from build123d import *

# Parameters (mm, degrees)
F0_R     = 3.203715
F1_DEPTH = 3
F2_DEPTH = 25.4
F3_DEPTH = 2
F5_DEPTH = 10


with BuildPart() as f1:
    # F0 (on Top) → F1 (new body)
    with BuildSketch(Plane.XY):
        with BuildLine():
            ThreePointArc((-11.680029, 20.96609), (-17.5, 21.857493), (-17.903305, 15.983481))
            ThreePointArc((-17.903305, 15.983481), (-23.978213, 1.022394), (-19.198874, -14.401501))
            ThreePointArc((-19.198874, -14.401501), (-18.823966, -15.285228), (-18.90402, -16.241848))
            Line((-18.90402, -16.241848), (-20.787271, -21.815403))
            ThreePointArc((-20.787271, -21.815403), (-24.589744, -23.697211), (-22.707936, -27.499683))
            Line((-22.707936, -27.499683), (-24.850231, -33.839886))
            ThreePointArc((-24.850231, -33.839886), (-24.445404, -36.549362), (-22.00809, -37.800219))
            Line((-22.00809, -37.800219), (-14.760585, -37.800219))
            ThreePointArc((-14.760585, -37.800219), (-11.760585, -40.800219), (-8.760585, -37.800219))
            Line((-8.760585, -37.800219), (8.760585, -37.800219))
            ThreePointArc((8.760585, -37.800219), (11.760585, -40.800219), (14.760585, -37.800219))
            Line((14.760585, -37.800219), (22.00809, -37.800219))
            ThreePointArc((22.00809, -37.800219), (24.445404, -36.549362), (24.850231, -33.839886))
            Line((24.850231, -33.839886), (22.707936, -27.499683))
            ThreePointArc((22.707936, -27.499683), (24.589744, -23.697211), (20.787271, -21.815403))
            Line((20.787271, -21.815403), (18.90402, -16.241848))
            ThreePointArc((18.90402, -16.241848), (18.823966, -15.285228), (19.198874, -14.401501))
            ThreePointArc((19.198874, -14.401501), (23.978213, 1.022394), (17.903305, 15.983481))
            ThreePointArc((17.903305, 15.983481), (17.5, 21.857493), (11.680029, 20.96609))
            ThreePointArc((11.680029, 20.96609), (0, 24), (-11.680029, 20.96609))
        make_face()
        with BuildLine():
            Line((0, -32.800219), (-15.040925, -32.800219))
            ThreePointArc((-15.040925, -32.800219), (-17.478239, -31.549362), (-17.883065, -28.839886))
            Line((-17.883065, -28.839886), (-12.493026, -12.88786))
            ThreePointArc((-12.493026, -12.88786), (-11.625772, -12.069632), (-10.462435, -12.330929))
            Line((-10.462435, -12.330929), (-7.587114, -14.800219))
            Line((-7.587114, -14.800219), (-3.793557, -14.800219))
            Line((-3.793557, -14.800219), (0, -14.800219))
            Line((0, -14.800219), (3.793557, -14.800219))
            Line((3.793557, -14.800219), (7.587114, -14.800219))
            Line((7.587114, -14.800219), (10.462435, -12.330929))
            ThreePointArc((10.462435, -12.330929), (11.625772, -12.069632), (12.493026, -12.88786))
            Line((12.493026, -12.88786), (17.883065, -28.839886))
            ThreePointArc((17.883065, -28.839886), (17.478239, -31.549362), (15.040925, -32.800219))
            Line((15.040925, -32.800219), (0, -32.800219))
        make_face(mode=Mode.SUBTRACT)
        with Locations((-18.755235, 0.000856)):
            Circle(F0_R, mode=Mode.SUBTRACT)
        with BuildLine():
            ThreePointArc((0, 9.424817), (6.525388, 10.328945), (12.559127, 12.973208))
            ThreePointArc((12.559127, 12.973208), (15.477463, 12.755317), (16.189543, 9.916814))
            Line((16.189543, 9.916814), (11.735012, -6.569164))
            ThreePointArc((11.735012, -6.569164), (10.311116, -7.677698), (8.852234, -6.615628))
            Line((8.852234, -6.615628), (-8.852234, -6.615628))
            ThreePointArc((-8.852234, -6.615628), (-10.311116, -7.677698), (-11.735012, -6.569164))
            Line((-11.735012, -6.569164), (-16.189543, 9.916814))
            ThreePointArc((-16.189543, 9.916814), (-15.477463, 12.755317), (-12.559127, 12.973208))
            ThreePointArc((-12.559127, 12.973208), (-6.525388, 10.328945), (0, 9.424817))
        make_face(mode=Mode.SUBTRACT)
        with Locations((18.755235, 0.000856)):
            Circle(F0_R, mode=Mode.SUBTRACT)
        with BuildLine():
            ThreePointArc((-17.883065, -28.839886), (-17.478239, -31.549362), (-15.040925, -32.800219))
            Line((-15.040925, -32.800219), (0, -32.800219))
            Line((0, -32.800219), (15.040925, -32.800219))
            ThreePointArc((15.040925, -32.800219), (17.478239, -31.549362), (17.883065, -28.839886))
            Line((17.883065, -28.839886), (12.493026, -12.88786))
            ThreePointArc((12.493026, -12.88786), (11.625772, -12.069632), (10.462435, -12.330929))
            Line((10.462435, -12.330929), (7.587114, -14.800219))
            Line((7.587114, -14.800219), (3.793557, -14.800219))
            Line((3.793557, -14.800219), (1.896779, -16.519575))
            Line((1.896779, -16.519575), (3.978112, -24.680085))
            Line((3.978112, -24.680085), (0, -29.158387))
            Line((0, -29.158387), (-3.978112, -24.680085))
            Line((-3.978112, -24.680085), (-1.896779, -16.519575))
            Line((-1.896779, -16.519575), (-3.793557, -14.800219))
            Line((-3.793557, -14.800219), (-7.587114, -14.800219))
            Line((-7.587114, -14.800219), (-10.462435, -12.330929))
            ThreePointArc((-10.462435, -12.330929), (-11.625772, -12.069632), (-12.493026, -12.88786))
            Line((-12.493026, -12.88786), (-17.883065, -28.839886))
        make_face()
        Polygon((0, -18.238932), (-1.896779, -16.519575), (-3.978112, -24.680085), (0, -29.158387), (3.978112, -24.680085), (1.896779, -16.519575), align=None)
        Polygon((0, -14.800219), (-3.793557, -14.800219), (-1.896779, -16.519575), (0, -18.238932), (1.896779, -16.519575), (3.793557, -14.800219), align=None)
        Polygon((-8.852234, -6.615628), (8.852234, -6.615628), (7.976763, -3.746212), (0, -3.746212), (-7.976763, -3.746212), align=None)
    extrude(amount=F1_DEPTH)

    # F0 (on Top) → F2 (cut)
    with BuildSketch(Plane.XY):
        with BuildLine():
            ThreePointArc((-17.883065, -28.839886), (-17.478239, -31.549362), (-15.040925, -32.800219))
            Line((-15.040925, -32.800219), (0, -32.800219))
            Line((0, -32.800219), (15.040925, -32.800219))
            ThreePointArc((15.040925, -32.800219), (17.478239, -31.549362), (17.883065, -28.839886))
            Line((17.883065, -28.839886), (12.493026, -12.88786))
            ThreePointArc((12.493026, -12.88786), (11.625772, -12.069632), (10.462435, -12.330929))
            Line((10.462435, -12.330929), (7.587114, -14.800219))
            Line((7.587114, -14.800219), (3.793557, -14.800219))
            Line((3.793557, -14.800219), (1.896779, -16.519575))
            Line((1.896779, -16.519575), (3.978112, -24.680085))
            Line((3.978112, -24.680085), (0, -29.158387))
            Line((0, -29.158387), (-3.978112, -24.680085))
            Line((-3.978112, -24.680085), (-1.896779, -16.519575))
            Line((-1.896779, -16.519575), (-3.793557, -14.800219))
            Line((-3.793557, -14.800219), (-7.587114, -14.800219))
            Line((-7.587114, -14.800219), (-10.462435, -12.330929))
            ThreePointArc((-10.462435, -12.330929), (-11.625772, -12.069632), (-12.493026, -12.88786))
            Line((-12.493026, -12.88786), (-17.883065, -28.839886))
        make_face()
    extrude(amount=F2_DEPTH, mode=Mode.SUBTRACT)

    # F0 (on Top) → F3 (join)
    with BuildSketch(Plane.XY):
        with BuildLine():
            ThreePointArc((-17.883065, -28.839886), (-17.478239, -31.549362), (-15.040925, -32.800219))
            Line((-15.040925, -32.800219), (0, -32.800219))
            Line((0, -32.800219), (15.040925, -32.800219))
            ThreePointArc((15.040925, -32.800219), (17.478239, -31.549362), (17.883065, -28.839886))
            Line((17.883065, -28.839886), (12.493026, -12.88786))
            ThreePointArc((12.493026, -12.88786), (11.625772, -12.069632), (10.462435, -12.330929))
            Line((10.462435, -12.330929), (7.587114, -14.800219))
            Line((7.587114, -14.800219), (3.793557, -14.800219))
            Line((3.793557, -14.800219), (1.896779, -16.519575))
            Line((1.896779, -16.519575), (3.978112, -24.680085))
            Line((3.978112, -24.680085), (0, -29.158387))
            Line((0, -29.158387), (-3.978112, -24.680085))
            Line((-3.978112, -24.680085), (-1.896779, -16.519575))
            Line((-1.896779, -16.519575), (-3.793557, -14.800219))
            Line((-3.793557, -14.800219), (-7.587114, -14.800219))
            Line((-7.587114, -14.800219), (-10.462435, -12.330929))
            ThreePointArc((-10.462435, -12.330929), (-11.625772, -12.069632), (-12.493026, -12.88786))
            Line((-12.493026, -12.88786), (-17.883065, -28.839886))
        make_face()
    extrude(amount=F3_DEPTH)

    # F4 (on Right) → F5 (cut, symmetric)
    with BuildSketch(Plane.YZ):
        Polygon((-3.716471, 3.089604), (-6.690737, 3.080773), (-3.710722, 0), align=None)
    extrude(amount=F5_DEPTH, both=True, mode=Mode.SUBTRACT)


solid = f1.part
Source: CAD feature listing. Evaluate the final solid. Frame: model axes, mm. A direction names the side the tool comes from. Coordinates: 2 decimals unless noted, no trailing zeros. Order: outer loops, then holes, each group sorted by start corner. A loop starts at its lowest first (then second) coordinate and runs counter-clockwise, first axis right, second up.
Item 1: First-contact query: P1, Ø1.5, axis at x = 17, z = 1.5, coming from the -Y side; P2, Ø1, axis at x = -14, z = 2.5, coming from the -Y side; P3, Ø1, axis at x = 1.5, z = 0.5, coming from the +Y side. Flat tips, straight axial feed; report the tip coordinate or a pass-through.
Output values:
P1: stops at y = -37.8
P2: stops at y = -40.24
P3: stops at y = 23.98
Item 2: Pull-direction query (X, two-part tool) for faces 5 (the face through (-2.8, -15.7, 2.5)), 6 (the face through (0, -8, 3)), 7 (the face through (23.794, -30.714, 1.479)); classes: pulls with the +X half, pulls with the -X half, needs draft (parallel to the pull), parting line crosses it, or undercut.
Output values:
face 5: undercut
face 6: needs draft
face 7: pulls with the +X half
Item 3: Material intervals for line 1 (Y direction, x = 9.5, z = 2.1); line 2 (X direction, y = -25, z = 2.5); line 3 (X direction, y = -7, z = 0.1), sorted ascending.
Output values:
line 1: y = -39.77 to -32.8, -13.16 to -7.45, 11.39 to 22.04
line 2: x = -24.73 to -16.59, -3.69 to 3.69, 16.59 to 24.73
line 3: x = -22.96 to -11.54, -9.03 to 9.03, 11.54 to 22.96
Item 4: Cut plane A-A (y = 7). Return loops of the section in (x, z).
Output values:
outline: (-22.96, 0) - (-15.4, 0) - (-15.4, 3) - (-22.96, 3) - close; (15.4, 0) - (22.96, 0) - (22.96, 3) - (15.4, 3) - close
Item 5: Cut plane B-B (x = 14). Return loops of the section in (y, z).
Output values:
outline: (-39.8, 0) - (1.81, 0) - (1.81, 3) - (-17.35, 3) - (-17.35, 2) - (-32.8, 2) - (-32.8, 3) - (-39.8, 3) - close; (13.34, 0) - (22.61, 0) - (22.61, 3) - (13.34, 3) - close
Item 6: Set-up query: faces 1 (the face through (18, -37.8, 1)), 2 (the face through (0, 24, 1)), 3 (the face through (13.993, 1.789, 1.479)), 4 (the face through (15.226, -20.976, 2.493)). Return all of +Z, -Z, +X, -X, +Y, -Y with unobstructed straight access to the full face (end or side cutting, diameter ignored); none if empty.
Output values:
face 1: +Z, -Z, +X, -Y
face 2: +Z, -Z, +Y
face 3: +Z, -Z
face 4: +Z
Item 7: Cut plane C-C (z = 0.5). Count the separate pieces of the cut face and the enclosed holes in it, plus the area to 3 significant figures.
Output values:
separate pieces: 1
enclosed holes: 3
area: 2,170 mm2
